Autodesk Inventor part; units mm, degrees
ref_plane "YZ Plane" through (0, 0, 0) normal (1, 0, 0) x (0, 1, 0)
ref_plane "XZ Plane" through (0, 0, 0) normal (0, 1, 0) x (-1, 0, 0)
ref_plane "XY Plane" through (0, 0, 0) normal (0, 0, 1) x (1, 0, 0)
sketch "Sketch1" plane through (0, 0, 0) normal (0, 0, 1) x (1, 0, 0)
  line L0 (55.5625, 0) -> (-55.5625, 0)
  line L1 (-55.5625, 0) -> (0, 76.2)
  line L2 (0, 76.2) -> (55.5625, 0)
  line L3 (-55.5625, 0) -> (55.5625, 0)
  line L4 (55.5625, 0) -> (55.5625, -127)
  line L5 (55.5625, -127) -> (-55.5625, -127)
  line L6 (-55.5625, -127) -> (-55.5625, 0)
  point P0 (0, 0)
  point P1 (0, 0)
  dimension "d0" = 111.125
  dimension "d1" = 76.2
  dimension "d14" = 127
extrude "Extrusion1" add sketch "Sketch1" along normal blind 6.35
sketch "Sketch2" plane through (0, 0, 6.35) normal (0, 0, 1) x (1, 0, 0)
  line L0 (-12.7, 6.35) -> (12.7, 6.35) construction
  line L1 (-55.5625, -127) -> (55.5625, -127) construction
  point P0 (0, 6.35)
  point P1 (0, 6.35)
  point P2 (0, 76.2)
  dimension "d6" = 25.4
  dimension "d15" = 133.35
hole "Hole1" at (-12.7, 6.35, 6.35) at (0, 6.35, 6.35) at (12.7, 6.35, 6.35) direction (0, 0, -1) diameter 5.1054 end through all
fillet "Fillet2" radius 6.35 5 edges at (-55.5625, 0, 3.175) (55.5625, 0, 3.175) (0, 76.2, 3.175) (-55.5625, -127, 3.175) (55.5625, -127, 3.175)
sketch "Sketch3" plane through (0, 0, 6.35) normal (0, 0, 1) x (1, 0, 0)
  arc A0 (49.2125, -127) -> (55.5625, -120.65) centre (49.2125, -120.65) ccw construction
  line L0 (55.5625, -120.65) -> (55.5625, -2.0693) construction
  arc A1 (55.5625, -2.0693) -> (54.3433, 1.672) centre (49.2125, -2.0693) ccw construction
  line L1 (54.3433, 1.672) -> (5.1308, 69.1634) construction
  arc A2 (5.1308, 69.1634) -> (-5.1308, 69.1634) centre (0, 65.4222) ccw construction
  line L2 (-5.1308, 69.1634) -> (-54.3433, 1.672) construction
  arc A3 (-54.3433, 1.672) -> (-55.5625, -2.0693) centre (-49.2125, -2.0693) ccw construction
  line L3 (-55.5625, -2.0693) -> (-55.5625, -120.65) construction
  arc A4 (-55.5625, -120.65) -> (-49.2125, -127) centre (-49.2125, -120.65) ccw construction
  line L4 (-49.2125, -127) -> (49.2125, -127) construction
  circle A5 centre (0, 6.35) radius 2.5527 construction
  circle A6 centre (-12.7, 6.35) radius 2.5527 construction
  circle A7 centre (12.7, 6.35) radius 2.5527 construction
  line L5 (0, 31.75) -> (-30.7945, 0.9555) construction
  line L6 (0, 31.75) -> (30.7945, 0.9555) construction
  point P0 (0, 0)
  dimension "d17" = 25.4
sketch "Sketch4" plane through (0, 0, 6.35) normal (0, 0, 1) x (1, 0, 0)
  arc A0 (49.2125, -127) -> (55.5625, -120.65) centre (49.2125, -120.65) ccw construction
  line L0 (55.5625, -120.65) -> (55.5625, -2.0693) construction
  arc A1 (55.5625, -2.0693) -> (54.3433, 1.672) centre (49.2125, -2.0693) ccw construction
  line L1 (54.3433, 1.672) -> (5.1308, 69.1634) construction
  arc A2 (5.1308, 69.1634) -> (-5.1308, 69.1634) centre (0, 65.4222) ccw construction
  line L2 (-5.1308, 69.1634) -> (-54.3433, 1.672) construction
  arc A3 (-54.3433, 1.672) -> (-55.5625, -2.0693) centre (-49.2125, -2.0693) ccw construction
  line L3 (-55.5625, -2.0693) -> (-55.5625, -120.65) construction
  arc A4 (-55.5625, -120.65) -> (-49.2125, -127) centre (-49.2125, -120.65) ccw construction
  line L4 (-49.2125, -127) -> (49.2125, -127) construction
  circle A5 centre (0, 6.35) radius 2.5527 construction
  circle A6 centre (-12.7, 6.35) radius 2.5527 construction
  circle A7 centre (12.7, 6.35) radius 2.5527 construction
  point P0 (0, 0)
  point P1 (-12.7, -101.6)
  point P2 (-12.7, -76.2)
  point P3 (-19.05, -47.625)
  point P4 (-19.05, -6.35)
  dimension "d24" = 12.7
  dimension "d25" = 19.05
  dimension "d26" = 53.975
  dimension "d27" = 19.05
  dimension "d28" = 12.7
  dimension "d29" = 82.55
  dimension "d30" = 107.95
hole "Hole2" at (-12.7, -101.6, 6.35) at (-12.7, -76.2, 6.35) at (-19.05, -47.625, 6.35) at (-19.05, -6.35, 6.35) direction (0, 0, -1) diameter 9.525 end through all
mirror "Mirror1" about plane through (0, 0, 0) normal (1, 0, 0) of "Hole2"
sketch "Sketch5" plane through (0, 0, 6.35) normal (0, 0, 1) x (1, 0, 0)
  circle A0 centre (-76.2, -73.025) radius 16.6688 construction
  circle A1 centre (76.2, -73.025) radius 16.6688 construction
  line L0 (-76.2, -73.025) -> (76.2, -73.025) construction
  line L1 (-49.2125, -127) -> (49.2125, -127) construction
  circle A2 centre (-76.2, -73.025) radius 23.0187 construction
  circle A3 centre (76.2, -73.025) radius 23.0187 construction
  line L2 (0, -127) -> (-104.775, -127)
  line L3 (0, -127) -> (104.775, -127)
  circle A4 centre (19.05, -47.625) radius 4.7625 construction
  circle A5 centre (19.05, -6.35) radius 4.7625 construction
  circle A6 centre (12.7, -76.2) radius 4.7625 construction
  circle A7 centre (12.7, -101.6) radius 4.7625 construction
  circle A8 centre (-19.05, -47.625) radius 4.7625 construction
  circle A9 centre (-12.7, -101.6) radius 4.7625 construction
  circle A10 centre (-12.7, -76.2) radius 4.7625 construction
  circle A11 centre (-19.05, -6.35) radius 4.7625 construction
  arc A12 (49.2125, -127) -> (55.5625, -120.65) centre (49.2125, -120.65) ccw
  line L4 (55.5625, -120.65) -> (55.5625, -2.0693)
  arc A13 (55.5625, -2.0693) -> (54.3433, 1.672) centre (49.2125, -2.0693) ccw construction
  line L5 (54.3433, 1.672) -> (5.1308, 69.1634) construction
  arc A14 (5.1308, 69.1634) -> (-5.1308, 69.1634) centre (0, 65.4222) ccw construction
  line L6 (-5.1308, 69.1634) -> (-54.3433, 1.672) construction
  arc A15 (-54.3433, 1.672) -> (-55.5625, -2.0693) centre (-49.2125, -2.0693) ccw construction
  line L7 (-55.5625, -2.0693) -> (-55.5625, -120.65)
  arc A16 (-55.5625, -120.65) -> (-49.2125, -127) centre (-49.2125, -120.65) ccw
  line L8 (-49.2125, -127) -> (49.2125, -127) construction
  circle A17 centre (0, 6.35) radius 2.5527 construction
  circle A18 centre (-12.7, 6.35) radius 2.5527 construction
  circle A19 centre (12.7, 6.35) radius 2.5527 construction
  arc A20 (-99.2187, -73.025) -> (-55.5625, -83.2209) centre (-76.2, -73.025) ccw
  line L9 (55.5625, -120.65) -> (55.5625, -2.0693) construction
  arc A21 (55.5625, -83.2209) -> (99.2188, -73.025) centre (76.2, -73.025) ccw
  line L10 (-104.775, -127) -> (-104.775, -73.025)
  line L11 (104.775, -127) -> (104.775, -73.025)
  line L12 (-104.775, -73.025) -> (-99.2187, -73.025)
  line L13 (99.2188, -73.025) -> (104.775, -73.025)
  point P0 (0, 0)
  point P1 (0, -73.025)
  dimension "d40" = 152.4
  dimension "d41" = 53.975
  dimension "d42" = 33.3375
  dimension "d43" = 6.35
  dimension "d46" = 104.775
extrude "Extrusion3" add sketch "Sketch5" against normal up to surface (6.35 mm away)
fillet "Fillet3" radius 3.175 8 edges at (-104.775, -73.025, 3.175) (-99.2187, -73.025, 3.175) (-55.5625, -83.2209, 3.175) (55.5625, -83.2209, 3.175) (99.2188, -73.025, 3.175) (104.775, -73.025, 3.175) (-104.775, -127, 3.175) (104.775, -127, 3.175)
properties part number "CL7-017" material "Polycarbonate, Smoke"
Check sheet for the modelled part. Datum: model origin and axes. Units: mm. Coordinates: 2 decimals unless noted, no trailing zeros. Loops run counter-clockwise (first coordinate to the right, second up) from the corner with the lowest first, then second, coordinate; pieces in that order, holes last.
1) Gauge pin test, flat ends, axial feed: pin 1 (2 mm diameter, centred on x = -31, z = 3.5, fed in from +Y); pin 2 (1 mm diameter, centred on y = 24, z = 5, fed in from -X); pin 3 (1.5 mm diameter, centred on y = -74, z = 3.5, fed in from +X). Record the tip position at first contact, or that the pin passes through.
2) Sectioned sample at B-B (x = 0). Record the boundary of the cut face in (y, z).
3) Sectioned sample at D-D (x = -21.5). Record the boundary of the cut face in (y, z), and give its area (3 significant figures).
4) Sectioned sample at C-C (z = 3.25). Count the separate pieces of the cut face and the enclosed holes in it, and give its area (3 significant figures).
5) Material ranges on probe 1 along X at (y, z) = (-76.2, 3.5); probe 2 along Y at (x, z) = (12.7, 4.25); probe 3 along Y at (x, z) = (-14, 5.5), recorded low to high.
6) Release check for a two-part mould opening along Y. For faces 1 (the face through (-104.775, -102, 3)), 2 (the face through (-79.435, -95.815, 3.219)), 3 (the face through (-9.8, -97.82, 3.13)) record: released by +Y, released by -Y, zero draft, split by the parting line, or undercut.
7) Sectioned sample at A-A (y = -6.35). Record the boundary of the cut face in (x, z), and give its area (3 significant figures).
Check sheet entries:
1. pin 1: stops at y = 35.06
1. pin 2: stops at x = -38.43
1. pin 3: stops at x = 55.56
2. outline: (-127, 0) - (3.8, 0) - (3.8, 6.35) - (-127, 6.35) - close; (8.9, 0) - (71.77, 0) - (71.77, 6.35) - (8.9, 6.35) - close
3. outline: (-127, 0) - (-51.71, 0) - (-51.71, 6.35) - (-127, 6.35) - close; (-43.54, 0) - (-10.43, 0) - (-10.43, 6.35) - (-43.54, 6.35) - close; (-2.27, 0) - (46.71, 0) - (46.71, 6.35) - (-2.27, 6.35) - close
3. area: 999 mm2
4. separate pieces: 1
4. enclosed holes: 11
4. area: 21,300 mm2
5. probe 1: x = -55.56 to -17.46, -7.94 to 7.94, 17.46 to 55.56
5. probe 2: y = -127 to -106.36, -96.84 to -80.96, -71.44 to 3.8, 8.9 to 58.78
5. probe 3: y = -127 to -106.18, -97.02 to -80.78, -71.62 to 4.15, 8.55 to 57
6. face 1: zero draft
6. face 2: released by +Y
6. face 3: undercut
7. outline: (-55.56, 0) - (-23.81, 0) - (-23.81, 6.35) - (-55.56, 6.35) - close; (-14.29, 0) - (14.29, 0) - (14.29, 6.35) - (-14.29, 6.35) - close; (23.81, 0) - (55.56, 0) - (55.56, 6.35) - (23.81, 6.35) - close
7. area: 585 mm2
